from build123d import *

# Parameters (mm, degrees)
SKETCH1_W               = 120
SKETCH1_H               = 31.25
BOSS_EXTRUDE1_DEPTH     = 7
SKETCH2_W               = 120
SKETCH2_H               = 4
SKETCH2_H_2             = 2
BOSS_EXTRUDE2_DEPTH     = 8
CUT_EXTRUDE1_DEPTH      = 125.260059955
CUT_EXTRUDE1_DEPTH_BACK = 125.260059955
SKETCH3_W               = 102
SKETCH3_H               = 8
SKETCH3_H_2             = 3.5
CUT_EXTRUDE3_REACH      = 126.906
SKETCH6_W               = 5
SKETCH6_H               = 2
SKETCH4_W               = 3
SKETCH4_H               = 8.090611825
SKETCH4_H_2             = 10.659388175
CUT_EXTRUDE4_DEPTH      = 5
SKETCH5_W               = 3
SKETCH5_H               = 8.0580149
SKETCH5_H_2             = 11.6919851
BOSS_EXTRUDE3_DEPTH     = 5


with BuildPart() as part:
    # Sketch1 → Boss-Extrude1 (new body)
    with BuildSketch(Plane.XY):
        with Locations((60, 15.625)):
            Rectangle(SKETCH1_W, SKETCH1_H)
    extrude(amount=BOSS_EXTRUDE1_DEPTH)

    # Sketch2 → Boss-Extrude2 (add)
    with BuildSketch(Plane.XY.offset(7)):
        with Locations((60, 25.6)):
            Rectangle(SKETCH2_W, SKETCH2_H)
        with Locations((60, 1)):
            Rectangle(SKETCH2_W, SKETCH2_H_2)
    extrude(amount=BOSS_EXTRUDE2_DEPTH)

    # Sketch3 → Cut-Extrude1 (cut, two sides: drawn at the far end of the back side and taken through both)
    with BuildSketch(Plane.XY.offset(7).offset(-CUT_EXTRUDE1_DEPTH_BACK)):
        with Locations((61, 11.1)):
            Rectangle(SKETCH3_W, SKETCH3_H)
        with Locations((61, 21.85)):
            Rectangle(SKETCH3_W, SKETCH3_H_2)
    extrude(amount=CUT_EXTRUDE1_DEPTH + CUT_EXTRUDE1_DEPTH_BACK, mode=Mode.SUBTRACT)

    # Sketch6 → Cut-Extrude3 (cut, up to next)
    with BuildSketch(Plane.ZY, mode=Mode.PRIVATE) as cut_extrude3_sk1:
        with Locations((12.5, 1)):
            Rectangle(SKETCH6_W, SKETCH6_H)
    cut_extrude3_tool1 = extrude(cut_extrude3_sk1.sketch, amount=-CUT_EXTRUDE3_REACH, mode=Mode.PRIVATE) & part.part
    add(cut_extrude3_tool1.solids().sort_by_distance((0, 1, 12.5))[0], mode=Mode.SUBTRACT)

    # Sketch4 → Cut-Extrude4 (cut)
    with BuildSketch(Plane.ZY):
        with Locations((3.5, 24.204694088)):
            Rectangle(SKETCH4_W, SKETCH4_H)
        with Locations((3.5, 8.829694088)):
            Rectangle(SKETCH4_W, SKETCH4_H_2)
    extrude(amount=-CUT_EXTRUDE4_DEPTH, mode=Mode.SUBTRACT)

    # Sketch5 → Boss-Extrude3 (add)
    with BuildSketch(Plane(origin=(120, 0, 0), x_dir=(0, 0, -1), z_dir=(1, 0, 0))):
        with Locations((-3.5, 24.22099255)):
            Rectangle(SKETCH5_W, SKETCH5_H)
        with Locations((-3.5, 9.34599255)):
            Rectangle(SKETCH5_W, SKETCH5_H_2)
    extrude(amount=BOSS_EXTRUDE3_DEPTH)


solid = part.part
Read the model definition and answer for the solid it produces. Units are mm, in the model's axes. A direction names the side the tool comes from. Coordinates: 2 decimals unless noted, no trailing zeros. Order: outer loops, then holes, each group sorted by start corner. A loop starts at its lowest first (then second) coordinate and runs counter-clockwise, first axis right, second up. Notation, with made-up numbers: M 49.5,-22 L 69.5,-22 A38 cw 69.5,16 Z; hole C -19.5,39 d11. An arc over 180 degrees is marked long. Put each result on its own line as item: value. Start each with the question number.
Item 1: Given pin 1 Ø4 at (x, y) = (123.5, 6.5) entering from -Z; pin 2 Ø4 at (x, z) = (64.5, 10.5) entering from +Y; pin 3 Ø2 at (y, z) = (10.5, 3.5) entering from -X; pin 4 Ø2 at (x, y) = (82, 9) entering from -Z, each flat-ended and moving along its own axis, determine where each tip first touches the part or whether it passes through.
Item 2: Section B-B, the plane x = 38.5 is taken. Determine the outline of the cut face in (y, z).
Item 3: The mould has two halves that part along Z. Classify faces 6 (the face through (59, 0, 5)), 7 (the face through (2, 24, 5)), 8 (the face through (59, 26, 15)): +Z half, -Z half, draft (parallel to the pull), parting line (faces both ways), or undercut.
Item 4: For faces 1 (the face through (59, 1, 10)), 2 (the face through (122, 24, 5)), 3 (the face through (5, 9, 3)), 4 (the face through (122, 24, 2)), 5 (the face through (60, 20.1, 3)), determine the directions among +Z, -Z, +X, -X, +Y, -Y from which every point of the face is accessible in a straight line to the end or side of a thin tool.
Item 5: Section D-D, the plane x = 115.5 is taken. Determine the outline of the cut face in (y, z), plus the area to 3 significant figures.
Item 6: Section A-A, the plane y = 9.5 is taken. Determine the outline of the cut face in (x, z).
Item 7: Consider probe 1 along Y at (x, z) = (82, 3.5); probe 2 along Y at (x, z) = (39, 8.25); probe 3 along X at (y, z) = (10, 4.25). Determine where each line is inside the solid, lowest interval first. Write a range as [from, to].
Item 8: Section C-C, the plane z = 8.5 is taken. Determine the outline of the cut face in (x, y).
Computed:
1. pin 1: stops at z = 2
1. pin 2: stops at y = 27.6
1. pin 3: stops at x = 5
1. pin 4: passes through
2. outline: M 0,0 L 7.1,0 L 7.1,7 L 2,7 L 2,10 L 0,10 Z; M 15.1,0 L 20.1,0 L 20.1,7 L 15.1,7 Z; M 23.6,0 L 31.25,0 L 31.25,7 L 27.6,7 L 27.6,15 L 23.6,15 Z
3. face 6: draft
3. face 7: undercut
3. face 8: +Z half
4. face 1: +Z, +X, -X, -Y
4. face 2: +Z, +X, +Y, -Y
4. face 3: -X
4. face 4: -Z, +X, +Y, -Y
4. face 5: +Z, -Z
5. outline: M 0,0 L 31.25,0 L 31.25,7 L 27.6,7 L 27.6,15 L 23.6,15 L 23.6,7 L 2,7 L 2,10 L 0,10 Z
5. area: 257 mm2
6. outline: M 0,0 L 10,0 L 10,7 L 0,7 L 0,5 L 5,5 L 5,2 L 0,2 Z; M 112,0 L 120,0 L 120,2 L 125,2 L 125,5 L 120,5 L 120,7 L 112,7 Z
7. probe 1: y = [0, 7.1], [15.1, 20.1], [23.6, 31.25]
7. probe 2: y = [0, 2], [23.6, 27.6]
7. probe 3: x = [5, 10], [112, 125]
8. outline: M 0,0 L 120,0 L 120,2 L 0,2 Z; M 0,23.6 L 120,23.6 L 120,27.6 L 0,27.6 Z
